```python
from build123d import *

# Parameters (mm, degrees)
SKETCH_1_W                   = 40
SKETCH_1_H                   = 39
EXTRUDE_1_DEPTH              = 20
SKETCH_2_W                   = 20
SKETCH_2_H                   = 1
EXTRUDE_2_DEPTH              = 7
SKETCH_3_W                   = 20
SKETCH_3_H                   = 1
EXTRUDE_3_DEPTH              = 7
SKETCH_5_R                   = 2
CUT_EXTRUDE_1_DEPTH          = 46.716517803
SKETCH_6_R                   = 2
CUT_EXTRUDE_2_DEPTH          = 46.716517803
SKETCH_7_R                   = 8.045118309
EXTRUDE_4_DEPTH              = 1
SKETCH_8_R                   = 6.323674856
EXTRUDE_5_DEPTH              = 1
SKETCH_9_R                   = 3
EXTRUDE_6_DEPTH              = 3
HOLE_WIZARD_M3_1_D           = 2.5
HOLE_WIZARD_M3_1_DEPTH       = 14.5
HOLE_WIZARD_M3_1_CSINK_D     = 3.05
HOLE_WIZARD_M3_1_CSINK_ANGLE = 90
HOLE_WIZARD_M3_1_TIP         = 0.751075774


with BuildPart() as part:
    # 草图1 → 凸台-拉伸1 (new body)
    with BuildSketch(Plane.XY):
        Rectangle(SKETCH_1_W, SKETCH_1_H)
    extrude(amount=EXTRUDE_1_DEPTH)

    # 草图2 → 凸台-拉伸2 (add)
    with BuildSketch(Plane.ZY.offset(20)):
        with Locations((10, 11)):
            Rectangle(SKETCH_2_W, SKETCH_2_H)
    extrude(amount=EXTRUDE_2_DEPTH)

    # 草图3 → 凸台-拉伸3 (add)
    with BuildSketch(Plane(origin=(20, 0, 0), x_dir=(0, 0, -1), z_dir=(1, 0, 0))):
        with Locations((-10, 11)):
            Rectangle(SKETCH_3_W, SKETCH_3_H)
    extrude(amount=EXTRUDE_3_DEPTH)

    # 草图5 → 切除-拉伸1 (cut, through all)
    with BuildSketch(Plane(origin=(0, 11.5, 0), x_dir=(1, 0, 0), z_dir=(0, 1, 0))):
        with Locations(Location((-24, -5.073781131, 0), (0, 0, 270))):
            Circle(SKETCH_5_R)
        with Locations(Location((-24, -14.926218869, 0), (0, 0, 270))):
            Circle(SKETCH_5_R)
    extrude(amount=-CUT_EXTRUDE_1_DEPTH, mode=Mode.SUBTRACT)

    # 草图6 → 切除-拉伸2 (cut, through all)
    with BuildSketch(Plane(origin=(0, 11.5, 0), x_dir=(1, 0, 0), z_dir=(0, 1, 0))):
        with Locations(Location((24, -5, 0), (0, 0, 180))):
            Circle(SKETCH_6_R)
        with Locations(Location((24, -15, 0), (0, 0, 180))):
            Circle(SKETCH_6_R)
    extrude(amount=-CUT_EXTRUDE_2_DEPTH, mode=Mode.SUBTRACT)

    # 草图7 → 凸台-拉伸4 (add)
    with BuildSketch(Plane(origin=(0, 19.5, 0), x_dir=(1, 0, 0), z_dir=(0, 1, 0))):
        with Locations(Location((-10, -10, 0), (0, 0, 90))):
            Circle(SKETCH_7_R)
    extrude(amount=EXTRUDE_4_DEPTH)

    # 草图8 → 凸台-拉伸5 (add)
    with BuildSketch(Plane(origin=(0, 20.5, 0), x_dir=(1, 0, 0), z_dir=(0, 1, 0))):
        with Locations(Location((-10, -10, 0), (0, 0, 270))):
            Circle(SKETCH_8_R)
    extrude(amount=EXTRUDE_5_DEPTH)

    # 草图9 → 凸台-拉伸6 (add)
    with BuildSketch(Plane(origin=(0, 21.5, 0), x_dir=(1, 0, 0), z_dir=(0, 1, 0))):
        with Locations(Location((-10, -10, 0), (0, 0, 270))):
            Circle(SKETCH_9_R)
    extrude(amount=EXTRUDE_6_DEPTH)

    # M3 螺纹孔1
    with Locations(Plane(origin=(-10.109547736, 24.5, 9.891000731), x_dir=(0, 0, 1), z_dir=(0, 1, 0))):
        with Locations((0, 0)):
            CounterSinkHole(HOLE_WIZARD_M3_1_D / 2, HOLE_WIZARD_M3_1_CSINK_D / 2, depth=HOLE_WIZARD_M3_1_DEPTH, counter_sink_angle=HOLE_WIZARD_M3_1_CSINK_ANGLE)
            with Locations((0, 0, -(HOLE_WIZARD_M3_1_DEPTH + HOLE_WIZARD_M3_1_TIP / 2))):  # 118° drill point
                Cone(0, HOLE_WIZARD_M3_1_D / 2, HOLE_WIZARD_M3_1_TIP, mode=Mode.SUBTRACT)


solid = part.part
```
Can you work these out from the model? Positions are in its coordinate system, mm. A direction names the side the tool comes from. Give positions to 0.01 mm unless a question says otherwise; leave off trailing zeros. Order: outer loops, then holes, each group sorted by start corner. A loop starts at its lowest first (then second) coordinate and runs counter-clockwise, first axis right, second up. Notation, with made-up numbers: M 7,13 L 22,13 A25 ccw 22,27 Z; hole C 69,67.25 d9. An arc over 180 degrees is marked long. Write item = value, one per line. Start each with the question number.
Q1. Suppose I cut it at D-D (y = -10.5). Write out the boundary of the cut face in (x, z).
Q2. Will these pins go through, and if not, where does the flat tip stop? pin 1 Ø5 at (y, z) = (-11, 14.5) entering from +X; pin 2 Ø12 at (x, z) = (18, 5) entering from +Y; pin 3 Ø5.5 at (x, z) = (23, 10) entering from +Y; pin 4 Ø2.5 at (x, z) = (24, 5) entering from -Y.
Q3. Suppose I cut it at C-C (x = -5). Write out the boundary of the cut face in (y, z), plus the area to 3 significant figures.
Q4. I need wall thicknesses on probe 1 along Z at (x, y) = (24, 11); probe 2 along Y at (x, z) = (2, 18); probe 3 along Y at (x, z) = (-12, 5.75). Which ranges of each line are inside material? Lowest first, please. Write a range as [from, to].
Q5. Suppose I cut it at B-B (z = 15). Write out the boundary of the cut face in (x, y), plus the area to 3 significant figures.
Q6. For faces 1 (the flat face through (-20, -5, 10)), 2 (the flat face through (20, -5, 10)), 3 (the cylindrical face through (-9.1, 22.98, 12.86)), 4 (the flat face through (23, 11.5, 10)), which set-ups out of +Z, -Z, +X, -X, +Y, -Y let a thin tool reach every point of the face, with its end or its side?
Q7. Suppose I cut it at A-A (x = 24). Write out the boundary of the cut face in (y, z), plus the area to 3 significant figures.
Check result:
q1.outline = M -20,0 L 20,0 L 20,20 L -20,20 Z
q2.pin_1 = 20
q2.pin_2 = 19.5
q2.pin_3 = 11.5
q2.pin_4 = through
q3.outline = M -19.5,0 L 19.5,0 L 19.5,3.7 L 20.5,3.7 L 20.5,6.13 L 21.5,6.13 L 21.5,13.87 L 20.5,13.87 L 20.5,16.3 L 19.5,16.3 L 19.5,20 L -19.5,20 Z
q3.area = 800 mm2
q4.probe_1 = [0, 3], [7, 13], [17, 20]
q4.probe_2 = [-19.5, 19.5]
q4.probe_3 = [-19.5, 21.5]
q5.outline = M -27,10.5 L -26,10.5 L -26,11.5 L -27,11.5 Z; M -22,10.5 L -20,10.5 L -20,-19.5 L 20,-19.5 L 20,10.5 L 22,10.5 L 22,11.5 L 20,11.5 L 20,19.5 L -3.7,19.5 L -3.7,20.5 L -6.13,20.5 L -6.13,21.5 L -13.87,21.5 L -13.87,20.5 L -16.3,20.5 L -16.3,19.5 L -20,19.5 L -20,11.5 L -22,11.5 Z; M 26,10.5 L 27,10.5 L 27,11.5 L 26,11.5 Z
q5.area = 1,590 mm2
q6.face_1 = +Z, -Z, -X, -Y
q6.face_2 = +Z, -Z, +X, -Y
q6.face_3 = +Y
q6.face_4 = +Z, -Z, +X, +Y
q7.outline = M 10.5,0 L 11.5,0 L 11.5,3 L 10.5,3 Z; M 10.5,7 L 11.5,7 L 11.5,13 L 10.5,13 Z; M 10.5,17 L 11.5,17 L 11.5,20 L 10.5,20 Z
q7.area = 12.0 mm2
